Could you check a few things on this drawing? It's one solid part, dimensions in mm from its lowest x, y, z. Round coordinates to 2 decimals unless told otherwise and drop trailing zeros. Order: outer loops, then holes, each group sorted by start corner. A loop starts at its lowest first (then second) coordinate and runs counter-clockwise, first axis right, second up. Notation, with made-up numbers: (40, 49.5) -> (45, 49.5) arc R20 ccw to (45, 67.5) -> close; hole circle Ø11 at (19.25, -21.75). An arc over 180 degrees is marked (long way). Use a Markdown table: item, result. Add a question column.
(1) If I drill on probe 1 along Z at (x, y) = (9.5, 1.45); probe 2 along X at (y, z) = (1.5, 23.5); probe 3 along X at (y, z) = (1.2, 52.5), over which ranges is the centre line in solid material (lowest first)?
(2) I want a section at C-C, the plane z = 26.5. Please give me the cut outline in (x, y), then the cut area to 3 significant figures.
(3) I'm going to push a flat-ended pin straight in: P1, Ø1.1, axis at x = 9.5, z = 23.5, coming from the +Y side. Where does the tip first touch, or does it pass through?
(4) I want a section at A-A, the plane z = 53. Please give me the cut outline in (x, y), then the cut area to 3 significant figures.
(5) I want a section at B-B, the plane x = 15.5. Please give me the cut outline in (y, z), then the cut area to 3 significant figures.
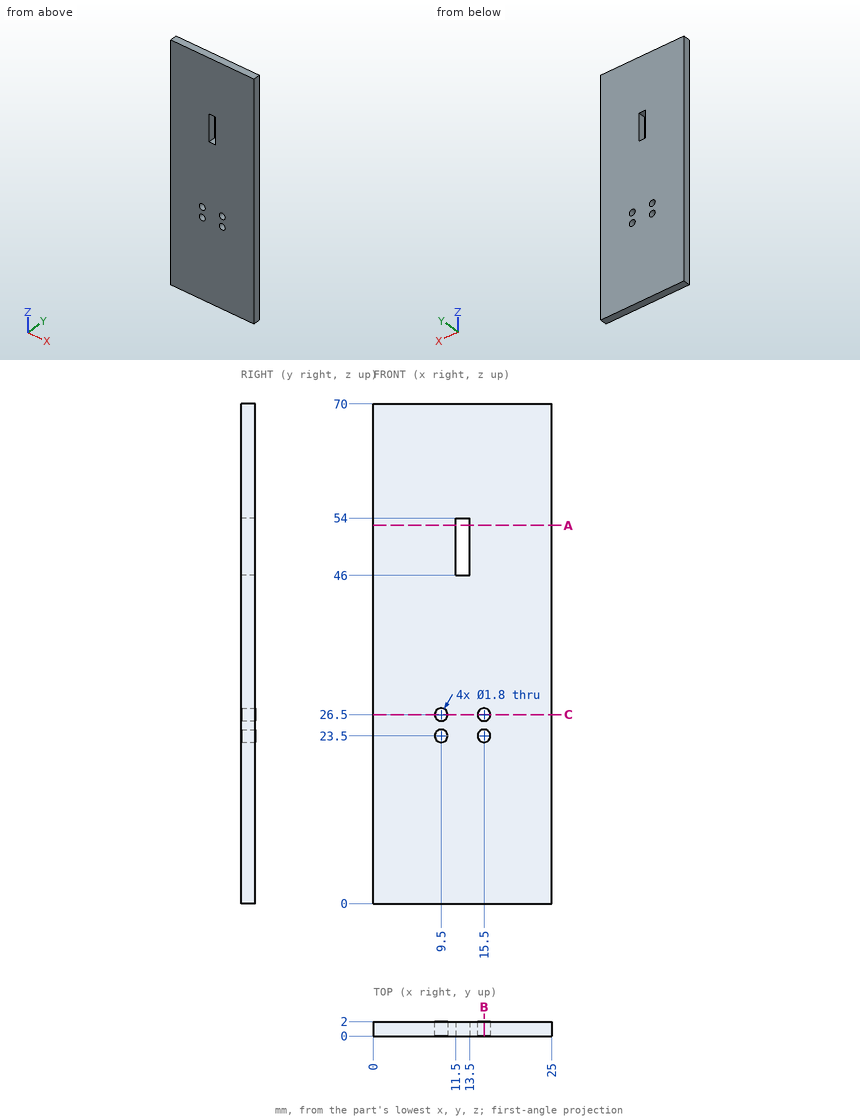
Taken from the geometry:
| question | item | result |
|---|---|---|
| 1 | probe 1 | z = 0 to 22.6, 24.4 to 25.6, 27.4 to 70 |
| 1 | probe 2 | x = 0 to 8.6, 10.4 to 14.6, 16.4 to 25 |
| 1 | probe 3 | x = 0 to 11.5, 13.5 to 25 |
| 2 | outline | (0, 0) -> (8.6, 0) -> (8.6, 2) -> (0, 2) -> close; (10.4, 0) -> (14.6, 0) -> (14.6, 2) -> (10.4, 2) -> close; (16.4, 0) -> (25, 0) -> (25, 2) -> (16.4, 2) -> close |
| 2 | area | 42.8 mm2 |
| 3 | P1 | passes through |
| 4 | outline | (0, 0) -> (11.5, 0) -> (11.5, 2) -> (0, 2) -> close; (13.5, 0) -> (25, 0) -> (25, 2) -> (13.5, 2) -> close |
| 4 | area | 46.0 mm2 |
| 5 | outline | (0, 0) -> (2, 0) -> (2, 22.6) -> (0, 22.6) -> close; (0, 24.4) -> (2, 24.4) -> (2, 25.6) -> (0, 25.6) -> close; (0, 27.4) -> (2, 27.4) -> (2, 70) -> (0, 70) -> close |
| 5 | area | 133 mm2 |
